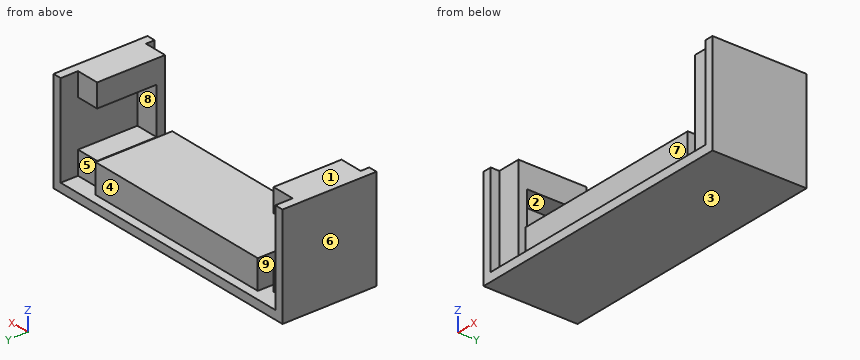
```python
from build123d import *

# Parameters (mm, degrees)
F0_W      = 609.6
F0_H      = 206.375
F1_DEPTH  = 19.05
F2_W      = 431.8
F2_H      = 168.275
F3_DEPTH  = 63.5
F4_W      = 19.05
F4_H      = 206.375
F5_DEPTH  = 203.2
F6_W      = 50.8
F6_H      = 130.175
F7_DEPTH  = 50.8
F8_W      = 130.175
F8_H      = 50.8
F9_DEPTH  = 50.8
F10_W     = 130.175
F10_H     = 50.8
F11_DEPTH = 50.8
F12_W     = 50.8
F12_H     = 203.2
F13_DEPTH = 19.05


with BuildPart() as f1:
    # F0 (on Top) → F1 (new body)
    with BuildSketch(Plane.XY):
        with Locations((304.8, 103.1875)):
            Rectangle(F0_W, F0_H)
    extrude(amount=F1_DEPTH)

    # F2 (on face) → F3 (join)
    with BuildSketch(Plane.XY.offset(19.05)):
        with Locations((304.8, 103.1875)):
            Rectangle(F2_W, F2_H)
    extrude(amount=F3_DEPTH)

    # F4 (on face) → F5 (join)
    with BuildSketch(Plane.XY.offset(19.05)):
        with Locations((9.525, 103.1875)):
            Rectangle(F4_W, F4_H)
        with Locations((600.075, 103.1875)):
            Rectangle(F4_W, F4_H)
    extrude(amount=F5_DEPTH)

    # F6 (on face) → F7 (join)
    with BuildSketch(Plane.XY.offset(19.05)):
        with Locations((44.45, 103.1875)):
            Rectangle(F6_W, F6_H)
        with Locations((565.15, 103.1875)):
            Rectangle(F6_W, F6_H)
    extrude(amount=F7_DEPTH)

    # F8 (on face) → F9 (join)
    with BuildSketch(Plane.YZ.offset(19.05)):
        with Locations((103.1875, 196.85)):
            Rectangle(F8_W, F8_H)
    extrude(amount=F9_DEPTH)

    # F10 (on face) → F11 (join)
    with BuildSketch(Plane(origin=(590.55, 0, 0), x_dir=(0, -1, 0), z_dir=(-1, 0, 0))):
        with Locations((-103.1875, 196.85)):
            Rectangle(F10_W, F10_H)
    extrude(amount=F11_DEPTH)

    # F12 (on face) → F13 (join)
    with BuildSketch(Plane.XZ.offset(-38.1)):
        with Locations((44.45, 120.65)):
            Rectangle(F12_W, F12_H)
        with Locations((565.15, 120.65)):
            Rectangle(F12_W, F12_H)
    extrude(amount=F13_DEPTH)


solid = f1.part
```
Could you check a few things on this model? Use its own coordinates, in mm. Face numbers are marked on the shaded views. A direction names the side the tool comes from. Coordinates: 2 decimals unless noted, no trailing zeros. Write each loop counter-clockwise with the first axis right and the second up, starting at its lowest first coordinate (ties: lowest second). Pieces come first, ordered by that corner, then holes. Notation, with made-up numbers: (48.5, 33) -> (94.5, 33) arc R25 cw to (94.5, 64) -> close; hole circle Ø2 at (48.5, -24). An arc over 180 degrees is marked (long way). Return JSON: item names as keys, results as strings.
(1) Imagine slicing it at D-D, the plane z = 115.5. Please give me the cut outline in (x, y) (3 decimals).
Numbers:
{"outline": "(0, 0) -> (19.05, 0) -> (19.05, 19.05) -> (69.85, 19.05) -> (69.85, 38.1) -> (19.05, 38.1) -> (19.05, 206.375) -> (0, 206.375) -> close; (539.75, 19.05) -> (590.55, 19.05) -> (590.55, 0) -> (609.6, 0) -> (609.6, 206.375) -> (590.55, 206.375) -> (590.55, 38.1) -> (539.75, 38.1) -> close"}
(2) Which directions (+Z, -Z, +X, -X, +Y, -Y) give clear straight access to the entire face, cutting with the end or side of a thin tool? Please do the marked faces 5, 6, 7, 8 and 9.
Numbers:
{"face 5": "+Z, +Y", "face 6": "+Z, -Z, -X, +Y, -Y", "face 7": "+Z, -Y", "face 8": "+Y", "face 9": "+Z, +Y, -Y"}
(3) Imagine slicing it at A-A, the plane z = 193.5. Please give me the cut outline in (x, y) (3 decimals), then the cut area to 3 significant figures.
Numbers:
{"outline": "(0, 0) -> (19.05, 0) -> (19.05, 19.05) -> (69.85, 19.05) -> (69.85, 168.275) -> (19.05, 168.275) -> (19.05, 206.375) -> (0, 206.375) -> close; (539.75, 19.05) -> (590.55, 19.05) -> (590.55, 0) -> (609.6, 0) -> (609.6, 206.375) -> (590.55, 206.375) -> (590.55, 168.275) -> (539.75, 168.275) -> close", "area": "23,000 mm2"}
(4) Imagine slicing it at B-B, the plane x = 571.5. Please give me the cut outline in (y, z) (3 decimals).
Numbers:
{"outline": "(0, 0) -> (206.375, 0) -> (206.375, 19.05) -> (168.275, 19.05) -> (168.275, 69.85) -> (38.1, 69.85) -> (38.1, 171.45) -> (168.275, 171.45) -> (168.275, 222.25) -> (19.05, 222.25) -> (19.05, 19.05) -> (0, 19.05) -> close"}
(5) We'd pull the mould along Z, two halves only. Please class the marked faces 1, 2, 3 and 4: +Z half, -Z half, draft (parallel to the pull), parting line (faces both ways), or undercut.
Numbers:
{"face 1": "+Z half", "face 2": "undercut", "face 3": "-Z half", "face 4": "draft"}
(6) I'm going to push flat-ended pins straight in: pin 1 (1.5 mm diameter, centred on x = 144.5, z = 43, fed in from +Y) (3 decimals); pin 2 (8 mm diameter, centred on x = 449.5, y = 61, fed in from +Z). Where does each tip first touch, or does it pass through?
Numbers:
{"pin 1": "stops at y = 187.325", "pin 2": "stops at z = 82.55"}
(7) I need wall thicknesses on L1, parallel to X at y = 112, z = 27.5; L2, parallel to X at y = 173.5, z = 206; L3, parallel to X at y = 50, z = 182.5. Which ranges of each line are inside material? Lowest first, please.
Numbers:
{"L1": "x = 0 to 69.85, 88.9 to 520.7, 539.75 to 609.6", "L2": "x = 0 to 19.05, 590.55 to 609.6", "L3": "x = 0 to 69.85, 539.75 to 609.6"}
(8) Imagine slicing it at C-C, the plane y = 97. Please give me the cut outline in (x, z).
Numbers:
{"outline": "(0, 0) -> (609.6, 0) -> (609.6, 222.25) -> (539.75, 222.25) -> (539.75, 171.45) -> (590.55, 171.45) -> (590.55, 69.85) -> (539.75, 69.85) -> (539.75, 19.05) -> (520.7, 19.05) -> (520.7, 82.55) -> (88.9, 82.55) -> (88.9, 19.05) -> (69.85, 19.05) -> (69.85, 69.85) -> (19.05, 69.85) -> (19.05, 171.45) -> (69.85, 171.45) -> (69.85, 222.25) -> (0, 222.25) -> close"}
